The drawing under review shows one solid part. Ordinate dimensions are in mm from its lowest x, y, z. A direction names the side the tool comes from. Round coordinates to 2 decimals unless told otherwise and drop trailing zeros. Order: outer loops, then holes, each group sorted by start corner. A loop starts at its lowest first (then second) coordinate and runs counter-clockwise, first axis right, second up. Notation, with made-up numbers: M -39.75,-6.5 L 17.25,-6.5 A25 cw 17.25,12.5 Z; hole C 23.5,59.5 d5. An arc over 180 degrees is marked long. Use a Markdown table: item, result.
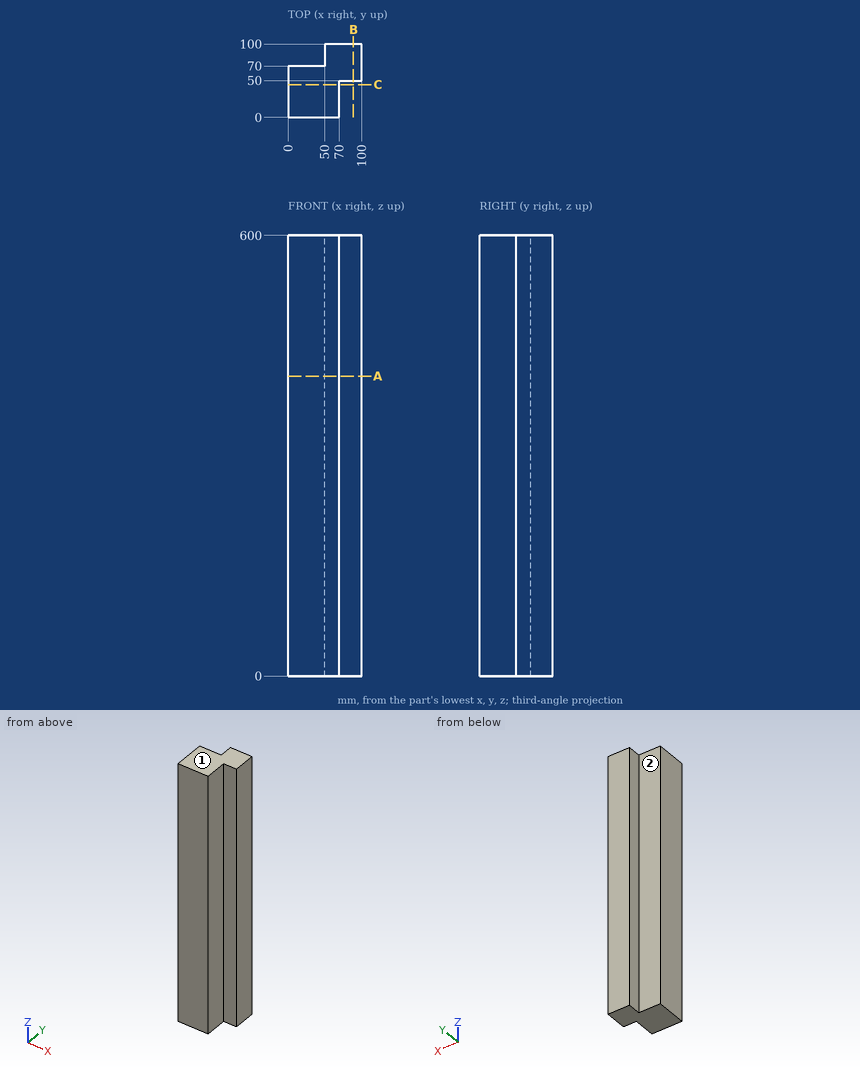
Q1. Machinability: for the marked faces 1 and 2, which of the approach directions +Z, -Z, +X, -X, +Y, -Y give a long, thin tool a straight path to every point of the face, cutting with its end or side? Answer none if there is none.
Determined:
| item | result |
|---|---|
| face 1 | +Z, +X, -X, +Y, -Y |
| face 2 | +Z, -Z, -X, +Y |
Q2. Add section B-B (x = 89). Write out the cut boundary in (y, z), then the cut area to 3 significant figures.
Determined:
| item | result |
|---|---|
| outline | M 50,0 L 100,0 L 100,600 L 50,600 Z |
| area | 30,000 mm^2 |
Q3. Wall thickness on line 1 along Y through (x, z) = (91.5, 168); line 2 along Y through (x, z) = (42.5, 507.5): over which ranges is each line inside the solid? List them lowest first. Write a range as [from, to].
Determined:
| item | result |
|---|---|
| line 1 | y = [50, 100] |
| line 2 | y = [0, 70] |
Q4. Add section A-A (z = 408.5). Write out the cut boundary in (x, y), then the cut area to 3 significant figures.
Determined:
| item | result |
|---|---|
| outline | M 0,0 L 70,0 L 70,50 L 100,50 L 100,100 L 50,100 L 50,70 L 0,70 Z |
| area | 7,000 mm^2 |
Q5. Clearance check with flat-ended pins moving along their axes: pin 1 (1 mm diameter, centred on x = 26, z = 227.5, fed in from -Y); pin 2 (1 mm diameter, centred on y = 73, z = 421, fed in from -X); pin 3 (15 mm diameter, centred on y = 14, z = 385, fed in from +X); pin 4 (24 mm diameter, centred on x = 83, z = 247, fed in from -Y). State where each tip first meets the part, or that it passes through.
Determined:
| item | result |
|---|---|
| pin 1 | stops at y = 0 |
| pin 2 | stops at x = 50 |
| pin 3 | stops at x = 70 |
| pin 4 | stops at y = 50 |
Q6. Add section C-C (y = 44.5). Write out the cut boundary in (x, z).
Determined:
| item | result |
|---|---|
| outline | M 0,0 L 70,0 L 70,600 L 0,600 Z |
